Source: CAD feature listing. Evaluate the final solid. Frame: model axes, mm. Give positions to 0.01 mm unless a question says otherwise; leave off trailing zeros. Order: outer loops, then holes, each group sorted by start corner. A loop starts at its lowest first (then second) coordinate and runs counter-clockwise, first axis right, second up. Notation, with made-up numbers: M 78.5,-27 L 92.5,-27 A23 ccw 92.5,5 Z; hole C 70.25,31.25 d4. An arc over 180 degrees is marked long. Answer as a JSON object with one key per item and string values. Group by question number.
1. Section query C-C (z = 16). Output: boundary loops of the cut face in (x, y), plus the area to 3 significant figures.
2. Section query A-A (x = 0). Output: boundary loops of the cut face in (y, z), plus the area to 3 significant figures.
3. Section query D-D (x = -527). Output: boundary loops of the cut face in (y, z).
4. Material intervals for L1, parallel to X at y = 345, z = 19; L2, parallel to X at y = 230, z = 2.5; L3, parallel to X at y = -8, z = 17.75, sorted ascending. Write a range as [from, to].
5. Section query B-B (y = -334.5). Output: boundary loops of the cut face in (x, z), plus the area to 3 significant figures.
6. Pin query (flat end, axial travel): P1, Ø2, axis at x = 453.5, y = -151.5, coming from the +Z side; P2, Ø12, axis at x = -309.5, z = 11.5, coming from the -Y side. Return the tip coordinate at first contact, or that it passes through.
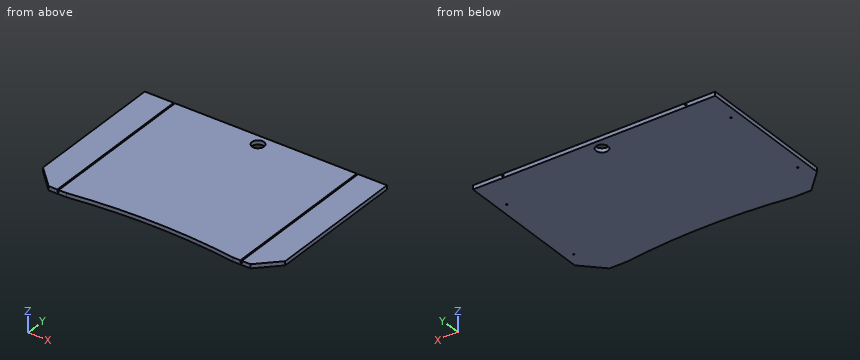
from build123d import *

# Parameters (mm, degrees)
SKETCH_R        = 30
PAD_DEPTH       = 20
SKETCH001_W     = 7
SKETCH001_H     = 942.511505
SKETCH001_H_2   = 1014.077607
POCKET_DEPTH    = 12
SKETCH002_R     = 3.7
POCKET001_DEPTH = 10
CHAMFER_SIZE    = 100


with BuildPart() as part:
    # Sketch → Pad (new body)
    with BuildSketch(Plane.XY):
        with BuildLine():
            Line((-600, 400), (600, 400))
            Line((600, 400), (600, -400))
            Line((600, -400), (412.1962, -400))
            ThreePointArc((412.1962, -400), (0, -371.547458), (-412.1962, -400))
            Line((-412.1962, -400), (-600, -400))
            Line((-600, -400), (-600, 400))
        make_face()
        with Locations((0, 345.880096)):
            Circle(SKETCH_R, mode=Mode.SUBTRACT)
    extrude(amount=PAD_DEPTH)

    # Sketch001 → Pocket (cut)
    with BuildSketch(Plane.XY.offset(20)):
        with Locations((-453.5, -23.519761)):
            Rectangle(SKETCH001_W, SKETCH001_H)
        with Locations((453.5, -39.674209)):
            Rectangle(SKETCH001_W, SKETCH001_H_2)
    extrude(amount=-POCKET_DEPTH, mode=Mode.SUBTRACT)

    # Sketch002 → Pocket001 (cut)
    with BuildSketch(Plane(origin=(0, 0, 0), x_dir=(1, 0, 0), z_dir=(0, 0, -1))):
        with Locations((-555, -230)):
            Circle(SKETCH002_R)
        with Locations((-555, 230)):
            Circle(SKETCH002_R)
        with Locations((555, 230)):
            Circle(SKETCH002_R)
        with Locations((555, -230)):
            Circle(SKETCH002_R)
    extrude(amount=-POCKET001_DEPTH, mode=Mode.SUBTRACT)

    # Chamfer
    chamfer_edges = [part.edges().sort_by_distance(p)[0] for p in [
        (-600, -400, 10),
        (600, -400, 10),
    ]]
    chamfer(chamfer_edges, length=CHAMFER_SIZE)


solid = part.part
Answer sheet:
{
 "1": {"outline": "M -600,-300 L -500,-400 L -457,-400 L -457,400 L -600,400 Z; M -450,-400 L -412.2,-400 A3000 cw 412.2,-400 L 450,-400 L 450,400 L -450,400 Z; M 457,-400 L 500,-400 L 600,-300 L 600,400 L 457,400 Z; hole C 0,345.88 d60", "area": "920,000 mm^2"},
 "2": {"outline": "M -371.55,0 L 315.88,0 L 315.88,20 L -371.55,20 Z; M 375.88,0 L 400,0 L 400,20 L 375.88,20 Z", "area": "14,200 mm^2"},
 "3": {"outline": "M -373,0 L 400,0 L 400,20 L -373,20 Z"},
 "4": {"L1": "[-600, -457], [-450, -29.99], [29.99, 450], [457, 600]", "L2": "[-600, -558.7], [-551.3, 551.3], [558.7, 600]", "L3": "[-600, -457], [-450, 450], [457, 600]"},
 "5": {"outline": "M -565.5,0 L 565.5,0 L 565.5,20 L 457,20 L 457,8 L 450,8 L 450,20 L -450,20 L -450,8 L -457,8 L -457,20 L -565.5,20 Z", "area": "22,500 mm^2"},
 "6": {"P1": "z = 8", "P2": "y = -388.18"}
}
